Build history of the part. All positions in model axes, mm. Face numbers are marked on the shaded views. A direction names the side the tool comes from. Round coordinates to 2 decimals unless told otherwise and drop trailing zeros. Write each loop counter-clockwise with the first axis right and the second up, starting at its lowest first coordinate (ties: lowest second). Pieces come first, ordered by that corner, then holes. Notation, with made-up numbers: (20, 26.5) - (53, 26.5) arc R23 cw to (53, 51.5) - close; hole circle Ø11 at (-24, -35.5). An arc over 180 degrees is marked (long way). One line per question, with ' | ' between items.
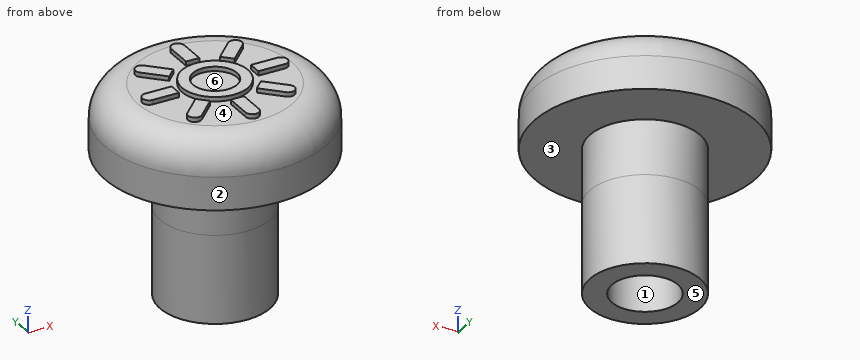
from build123d import *

# Parameters (mm, degrees)
SKETCH046_R        = 2.5
PAD023_DEPTH       = 2.5
SKETCH047_R        = 5
PAD024_DEPTH       = 3
FILLET003_R        = 1.5
SKETCH049_R        = 2.5
PAD025_DEPTH       = 4
SKETCH050_R        = 1.5
POCKET026_DEPTH    = 4
PAD053_DEPTH       = 0.2
SKETCH087_R        = 1.5
SKETCH087_R_2      = 1
PAD054_DEPTH       = 0.2
POLARPATTERN_COUNT = 8


with BuildPart() as part:
    # Sketch046 → Pad023 (new body)
    with BuildSketch(Plane(origin=(0, 0, 30), x_dir=(1, 0, 0), z_dir=(0, 0, -1))):
        with Locations((101, 55)):
            Circle(SKETCH046_R)
    extrude(amount=-PAD023_DEPTH)

    # Sketch047 (on Face3 of Pad023) → Pad024 (join)
    with BuildSketch(Plane.XY.offset(32.5)):
        with Locations((101, -55)):
            Circle(SKETCH047_R)
    extrude(amount=PAD024_DEPTH)

    # Fillet003
    fillet003_edges = [part.edges().sort_by_distance(p)[0] for p in [
        (96, -55, 35.5),
    ]]
    fillet(fillet003_edges, radius=FILLET003_R)

    # Sketch049 → Pad025 (join)
    with BuildSketch(Plane(origin=(0, 0, 30), x_dir=(1, 0, 0), z_dir=(0, 0, -1))):
        with Locations((101, 55)):
            Circle(SKETCH049_R)
    extrude(amount=PAD025_DEPTH)

    # Sketch050 (on Face17 of Pad025) → Pocket026 (cut)
    with BuildSketch(Plane(origin=(0, 0, 26), x_dir=(1, 0, 0), z_dir=(0, 0, -1))):
        with Locations((101, 55)):
            Circle(SKETCH050_R)
    extrude(amount=-POCKET026_DEPTH, mode=Mode.SUBTRACT)


with BuildPart() as part_1:
    # Body002 placement: moved
    add(part.part.moved(Location((75, 0, 0))))

    # Sketch086 (on Face4 of Clone001) → Pad053 (new body)
    with BuildSketch(Plane(origin=(176, -55, 35.5), x_dir=(1, 0, 0), z_dir=(0, 0, 1))):
        with BuildLine():
            Line((1.8, 0.3), (1.8, -0.3))
            Line((1.8, -0.3), (3, -0.3))
            ThreePointArc((3, -0.3), (3.3, 0), (3, 0.3))
            Line((1.8, 0.3), (3, 0.3))
        make_face()
    pad053 = extrude(amount=PAD053_DEPTH)

    # Sketch087 (on Face4 of Clone001) → Pad054 (join)
    with BuildSketch(Plane(origin=(176, -55, 35.5), x_dir=(1, 0, 0), z_dir=(0, 0, 1))):
        Circle(SKETCH087_R)
        Circle(SKETCH087_R_2, mode=Mode.SUBTRACT)
    extrude(amount=PAD054_DEPTH)

    # PolarPattern: Pad053 ×8 about axis
    polarpattern_axis = Axis((176, -55, 35.5), (0, 0, 1))
    for i in range(1, POLARPATTERN_COUNT):
        add(pad053.rotate(polarpattern_axis, i * 360 / POLARPATTERN_COUNT))


with BuildPart() as part_2:
    # Body011 placement: moved
    add(part_1.part.moved(Location((-89, 0, 0))))


solid = part_2.part
Q1. Saw through at D-D, the plane z = 33.75. List the corners of the cut face in (x, y).
Found:
outline: circle Ø10 at (87, -55)
Q2. Which spindle directions (+Z, -Z, +X, -X, +Y, -Y) get a long thin tool onto all of the face, cutting with end or side? Do the marked faces 5 and 6. Say none if no direction does.
Found:
face 5: -Z, +X, -X, +Y, -Y | face 6: +Z
Q3. Saw through at B-B, the plane z = 27. List the corners of the cut face in (x, y), then the cut area to 3 significant figures.
Found:
outline: circle Ø5 at (87, -55); hole circle Ø3 at (87, -55) | area: 12.6 mm^2
Q4. Drop flat-ended pins along their axis: pin 1 (1.5 mm diameter, centred on y = -53, z = 33, fed in from -X); pin 2 (3 mm diameter, centred on y = -57, z = 33.5, fed in from -X); pin 3 (1.8 mm diameter, centred on x = 87, y = -55, fed in from +Z). Give the stop position or say it passes through.
Found:
pin 1: x = 82.16 | pin 2: x = 82.03 | pin 3: z = 35.5
Q5. Drill centre lines: L1, parallel to Y at x = 87, z = 35.6; L2, parallel to Y at x = 87, z = 26.95; L3, parallel to Z at x = 86.5, y = -56.25. Where is each one in solid material? Low to high. Write a range as from..to.
Found:
L1: -58.3..-56.8, -56.5..-56, -54..-53.5, -53.2..-51.7 | L2: -57.5..-56.5, -53.5..-52.5 | L3: 30..35.7
Q6. Pull direction Y, two halves, no side cores. Call the marked faces 1, 2, 3 and 4: +Y half, -Y half, draft (parallel to the pull), parting line (faces both ways), or undercut.
Found:
face 1: undercut | face 2: parting line | face 3: draft | face 4: undercut
